For this review, take the finished solid that the model builds, in its own axes (mm). A direction names the side the tool comes from. Coordinates: 2 decimals unless noted, no trailing zeros. Loops run counter-clockwise (first coordinate to the right, second up) from the corner with the lowest first, then second, coordinate; pieces in that order, holes last. Notation, with made-up numbers: M 40,-4.5 L 77,-4.5 A26 ccw 77,18.5 Z; hole C 7,10.25 d10. An arc over 180 degrees is marked long. Put each result on its own line as item: value.
```python
from build123d import *

# Parameters (mm, degrees)
BOSS_EXTRUDE1_DEPTH     = 60
CUT_EXTRUDE1_DEPTH      = 10
FILLET1_R               = 10
SHELL1_T                = -2.4
CUT_EXTRUDE2_DEPTH      = 119.658164489
CUT_EXTRUDE2_DEPTH_BACK = 119.658164489
SKETCH3_R               = 1.65
SKETCH4_R               = 6
CUT_EXTRUDE3_DEPTH      = 119.658164667


with BuildPart() as part:
    # Sketch1 → Boss-Extrude1 (new body)
    with BuildSketch(Plane(origin=(0, 0, 0), x_dir=(1, 0, 0), z_dir=(0, 1, 0))):
        with BuildLine():
            Line((-10.4, 67), (10.4, 67))
            ThreePointArc((10.4, 67), (77.4, 0), (10.4, -67))
            Line((10.4, -67), (-10.4, -67))
            ThreePointArc((-10.4, -67), (-77.4, 0), (-10.4, 67))
        make_face()
    extrude(amount=BOSS_EXTRUDE1_DEPTH)

    # Sketch2 → Cut-Extrude1 (cut)
    with BuildSketch(Plane.XZ):
        Polygon((-91.251700072, 13), (-13, 13), (-13, 91.251700072), (13, 91.251700072), (13, 13), (91.251700072, 13), (91.251700072, -13), (13, -13), (13, -91.251700072), (-13, -91.251700072), (-13, -13), (-91.251700072, -13), align=None)
    extrude(amount=-CUT_EXTRUDE1_DEPTH, mode=Mode.SUBTRACT)

    # Fillet1
    fillet1_edges = [part.edges().sort_by_distance(p)[0] for p in [
        (-13, 5, 13),
        (13, 5, 13),
        (13, 5, -13),
        (-13, 5, -13),
    ]]
    fillet(fillet1_edges, radius=FILLET1_R)

    # Shell1
    shell1_openings = [part.faces().sort_by_distance(p)[0] for p in [
        (0, 60, 0),
    ]]
    offset(amount=SHELL1_T, openings=shell1_openings, kind=Kind.INTERSECTION)

    # Sketch3 → Cut-Extrude2 (cut, two sides: drawn at the far end of the back side and taken through both)
    with BuildSketch(Plane(origin=(0, 0, 0), x_dir=(0, 0, -1), z_dir=(1, 0, 0)).offset(-CUT_EXTRUDE2_DEPTH_BACK)):
        with Locations((0, 55)):
            Circle(SKETCH3_R)
    extrude(amount=CUT_EXTRUDE2_DEPTH + CUT_EXTRUDE2_DEPTH_BACK, mode=Mode.SUBTRACT)

    # Sketch4 → Cut-Extrude3 (cut, through all)
    with BuildSketch(Plane(origin=(0, 0, 0), x_dir=(0, 0, -1), z_dir=(1, 0, 0))):
        with Locations(Location((-45, 30, 0), (0, 0, 180))):
            Circle(SKETCH4_R)
    extrude(amount=CUT_EXTRUDE3_DEPTH, mode=Mode.SUBTRACT)


solid = part.part
```
(1) Add section A-A (y = 38). Write out the cut boundary in (x, z), plus the area to 3 significant figures.
Determined:
outline: M -10.4,-67 L 10.4,-67 A67 ccw 10.4,67 L -10.4,67 A67 ccw Z; hole M -10.4,-64.6 L 10.4,-64.6 A64.6 ccw 10.4,64.6 L -10.4,64.6 A64.6 ccw Z
area: 1,090 mm^2
(2) For pin 1 (1 mm diameter, centred on y = 25.5, z = -15.5, fed in from -X); pin 2 (2 mm diameter, centred on y = 45.5, z = -32, fed in from +X); pin 3 (3 mm diameter, centred on y = 2.5, z = -41.5, fed in from +X), all flat-tipped, find the tip position at first contact; note any pin that passes through.
Determined:
pin 1: stops at x = -75.7
pin 2: stops at x = 69.8
pin 3: stops at x = 64.15
(3) Add section B-B (z = 45). Write out the cut boundary in (x, y).
Determined:
outline: M -60.04,0 L -13,0 L -13,10 L 13,10 L 13,0 L 60.04,0 L 60.04,24 L 56.75,24 L 56.75,2.4 L 15.4,2.4 L 15.4,12.4 L -15.4,12.4 L -15.4,2.4 L -56.75,2.4 L -56.75,60 L -60.04,60 Z; M 56.75,36 L 60.04,36 L 60.04,60 L 56.75,60 Z
(4) Draft analysis for pull direction Y (two halves, no side actions). For faces 1 (the cylindrical face through (-76.206, 53.536, -0.761)), 2 (the flat face through (-15.4, 7, 43)), 3 (the flat face through (38, 2.4, -35)), state which applies: +Y half, -Y half, draft (parallel to the pull), parting line (faces both ways), or undercut.
Determined:
face 1: undercut
face 2: draft
face 3: +Y half
(5) Add section C-C (z = -58). Write out the cut boundary in (x, y).
Determined:
outline: M -43.94,0 L -13,0 L -13,10 L 13,10 L 13,0 L 43.94,0 L 43.94,60 L 38.85,60 L 38.85,2.4 L 15.4,2.4 L 15.4,12.4 L -15.4,12.4 L -15.4,2.4 L -38.85,2.4 L -38.85,60 L -43.94,60 Z
(6) Wall thickness on line 1 along Y through (x, z) = (-76, 0); line 2 along Z through (x, y) = (-1.5, 42); line 3 along Z through (x, y) = (40.5, 12): over which ranges is each line inside the solid? List them lowest first. Write a range as [from, to].
Determined:
line 1: y = [10, 53.35], [56.65, 60]
line 2: z = [-67, -64.6], [64.6, 67]
line 3: z = [-59.86, -57.16], [-15.4, 15.4], [57.16, 59.86]
(7) Add section D-D (x = 68.5). Write out the cut boundary in (y, z), plus the area to 3 significant figures.
Determined:
outline: M 0,-33.37 L 60,-33.37 L 60,-28.24 L 2.4,-28.24 L 2.4,-15.4 L 12.4,-15.4 L 12.4,15.4 L 2.4,15.4 L 2.4,28.24 L 60,28.24 L 60,33.37 L 0,33.37 L 0,13 L 10,13 L 10,-13 L 0,-13 Z
area: 799 mm^2
(8) Tool access review of faces 4 (the flat face through (38, 0, 34)), 5 (the flat face through (15.4, 7, 44)), 6 (the flat face through (-13, 5, -45)), 7 (the cylindrical face through (15.85, 5.07, -16.01)), 8 (the cylindrical face through (-77.384, 29.58, 1.473)): name each direction out of +Z, -Z, +X, -X, +Y, -Y from which nothing blocks a thin tool from reaching the whole face with its end or side.
Determined:
face 4: +Z, -Z, +X, -X, -Y
face 5: +Y
face 6: +Z, -Z, -Y
face 7: -Y
face 8: -X, +Y, -Y
